from build123d import *

# Parameters (mm, degrees)
SKETCH3_W                = 19.05
SKETCH3_H                = 19.05
SKETCH3_W_2              = 16.002
SKETCH3_H_2              = 16.002
BOSS_EXTRUDE1_DEPTH      = 25.4
BOSS_EXTRUDE1_DEPTH_BACK = 25.4
FILLET1_R                = 1.6002
SKETCH5_W                = 19.784949474
SKETCH5_H                = 25.4
CUT_EXTRUDE1_DEPTH       = 17.4625
SKETCH7_R                = 2.15265
CUT_EXTRUDE2_DEPTH       = 12.7
SKETCH6_R                = 2.15265
CUT_EXTRUDE3_DEPTH       = 2.524
SKETCH9_R                = 2.15265
CUT_EXTRUDE5_DEPTH       = 6.35
SKETCH10_R               = 2.15265
CUT_EXTRUDE6_DEPTH       = 20.05


with BuildPart() as part:
    # Sketch3 → Boss-Extrude1 (new body, two sides)
    with BuildSketch(Plane.XY) as boss_extrude1_sk:
        Rectangle(SKETCH3_W, SKETCH3_H)
        Rectangle(SKETCH3_W_2, SKETCH3_H_2, mode=Mode.SUBTRACT)
    extrude(amount=BOSS_EXTRUDE1_DEPTH)
    extrude(boss_extrude1_sk.sketch, amount=-BOSS_EXTRUDE1_DEPTH_BACK)

    # Fillet1
    fillet1_edges = [part.edges().sort_by_distance(p)[0] for p in [
        (8.001, -8.001, 0),
        (8.001, 8.001, 0),
        (-8.001, 8.001, 0),
        (-8.001, -8.001, 0),
        (9.525, -9.525, 0),
        (-9.525, -9.525, 0),
        (-9.525, 9.525, 0),
        (9.525, 9.525, 0),
    ]]
    fillet(fillet1_edges, radius=FILLET1_R)

    # Sketch5 → Cut-Extrude1 (cut)
    with BuildSketch(Plane(origin=(0, 9.525, 0), x_dir=(1, 0, 0), z_dir=(0, 1, 0))):
        with Locations((1.967674737, 0)):
            Rectangle(SKETCH5_W, SKETCH5_H)
    extrude(amount=-CUT_EXTRUDE1_DEPTH, mode=Mode.SUBTRACT)

    # Sketch7 → Cut-Extrude2 (cut)
    with BuildSketch(Plane(origin=(0, 9.525, 0), x_dir=(1, 0, 0), z_dir=(0, 1, 0))):
        with Locations((0, 19.05)):
            Circle(SKETCH7_R)
        with Locations((2.54, 0)):
            Circle(SKETCH7_R)
        with Locations((0, -19.05)):
            Circle(SKETCH7_R)
    extrude(amount=-CUT_EXTRUDE2_DEPTH, mode=Mode.SUBTRACT)

    # Sketch6 → Cut-Extrude3 (cut, through all)
    with BuildSketch(Plane(origin=(0, -8.001, 0), x_dir=(1, 0, 0), z_dir=(0, 1, 0))):
        with Locations((2.54, 0)):
            Circle(SKETCH6_R)
    extrude(amount=-CUT_EXTRUDE3_DEPTH, mode=Mode.SUBTRACT)

    # Sketch9 → Cut-Extrude5 (cut)
    with BuildSketch(Plane(origin=(9.525, 0, 0), x_dir=(0, 0, -1), z_dir=(1, 0, 0))):
        with Locations((-19.05, 0)):
            Circle(SKETCH9_R)
        with Locations((19.05, 0)):
            Circle(SKETCH9_R)
    extrude(amount=-CUT_EXTRUDE5_DEPTH, mode=Mode.SUBTRACT)

    # Sketch10 → Cut-Extrude6 (cut, through all)
    with BuildSketch(Plane(origin=(9.525, 0, 0), x_dir=(0, 0, -1), z_dir=(1, 0, 0))):
        with Locations((0, 2.54)):
            Circle(SKETCH10_R)
    extrude(amount=-CUT_EXTRUDE6_DEPTH, mode=Mode.SUBTRACT)


solid = part.part
The model under review builds one solid part; all positions refer to its coordinate system, in mm. A direction names the side the tool comes from. Give positions to 0.01 mm unless a question says otherwise; leave off trailing zeros. Loops run counter-clockwise (first coordinate to the right, second up) from the corner with the lowest first, then second, coordinate; pieces in that order, holes last. Notation, with made-up numbers: (52, 29.5) -> (94, 29.5) arc R21 cw to (94, 62.5) -> close; hole circle Ø7 at (4.25, 15.25). An arc over 180 degrees is marked (long way). Write each question's results on one line, items separated by ' | '.
1) Draft analysis for pull direction Y (two halves, no side actions). For faces 6 (the face through (-0.47, 8.77, 21.15)), 7 (the face through (9.07, -9.04, 0.36)), 8 (the face through (-8.001, 0, 0)), state which applies: pulls with the +Y half, pulls with the -Y half, needs draft (parallel to the pull), parting line crosses it, or undercut.
Conclusion:
face 6: needs draft | face 7: pulls with the -Y half | face 8: undercut
2) Take a section at D-D, the plane z = -19.05. Give the boundary of the cut face in (x, y) (3 decimals), plus the area to 3 significant figures.
Conclusion:
outline: (-9.525, -7.925) arc R1.6 ccw to (-7.925, -9.525) -> (7.925, -9.525) arc R1.6 ccw to (9.525, -7.925) -> (9.525, -2.153) -> (8.001, -2.153) -> (8.001, -6.401) arc R1.6 cw to (6.401, -8.001) -> (-6.401, -8.001) arc R1.6 cw to (-8.001, -6.401) -> (-8.001, 6.401) arc R1.6 cw to (-6.401, 8.001) -> (-2.153, 8.001) -> (-2.153, 9.525) -> (-7.925, 9.525) arc R1.6 ccw to (-9.525, 7.925) -> close; (2.153, 8.001) -> (6.401, 8.001) arc R1.6 cw to (8.001, 6.401) -> (8.001, 2.153) -> (9.525, 2.153) -> (9.525, 7.925) arc R1.6 ccw to (7.925, 9.525) -> (2.153, 9.525) -> close | area: 93.7 mm^2
3) Take a section at A-A, the plane x = -5.5. Give the boundary of the cut face in (y, z) (3 decimals).
Conclusion:
outline: (-9.525, -25.4) -> (-8.001, -25.4) -> (-8.001, 25.4) -> (-9.525, 25.4) -> close; (8.001, -25.4) -> (9.525, -25.4) -> (9.525, -12.7) -> (8.001, -12.7) -> close; (8.001, 12.7) -> (9.525, 12.7) -> (9.525, 25.4) -> (8.001, 25.4) -> close
4) Insertion check: pin 1 Ø7 at (y, z) = (2.54, 0) entering from +X; pin 2 Ø1.3 at (y, z) = (7.5, 0) entering from +X; pin 3 Ø10 at (x, z) = (1.5, -5) entering from +Y; pin 4 Ø0.8 at (x, y) = (-7.5, -7.5) entering from +Z. Each pin has a flat end and moves straight along its axis. Give the tip position at first contact, or say it passes through.
Conclusion:
pin 1: stops at x = -8 | pin 2: stops at x = -7.92 | pin 3: stops at y = -8 | pin 4: stops at z = 25.4
5) For line 1 along Z through (x, y) = (0, 9.2); line 2 along Y through (x, z) = (-3.5, -22) (3 decimals), list the stretches that pass through material, from the lowest coordinate up. Write a range as from..to.
Conclusion:
line 1: z = -25.4..-21.2, -16.9..-12.7, 12.7..16.9, 21.2..25.4 | line 2: y = -9.525..-8.001, 8.001..9.525
6) Take a section at C-C, the plane z = 14. Give the boundary of the cut face in (x, y) (3 decimals).
Conclusion:
outline: (-9.525, -7.925) arc R1.6 ccw to (-7.925, -9.525) -> (7.925, -9.525) arc R1.6 ccw to (9.525, -7.925) -> (9.525, 7.925) arc R1.6 ccw to (7.925, 9.525) -> (-7.925, 9.525) arc R1.6 ccw to (-9.525, 7.925) -> close; hole (-8.001, -6.401) arc R1.6 ccw to (-6.401, -8.001) -> (6.401, -8.001) arc R1.6 ccw to (8.001, -6.401) -> (8.001, 6.401) arc R1.6 ccw to (6.401, 8.001) -> (-6.401, 8.001) arc R1.6 ccw to (-8.001, 6.401) -> close
7) Tool access review of faces 1 (the face through (-7.7, -7.6, 12.7)), 2 (the face through (-1.9, 9.525, -17.5)), 3 (the face through (8.8, 0.1, 21.2)), 4 (the face through (8.001, 0, 22)), 5 (the face through (9.07, 9.04, -19.14)): name each direction out of +Z, -Z, +X, -X, +Y, -Y from which nothing blocks a thin tool from reaching the whole face with its end or side.
Conclusion:
face 1: +X, +Y | face 2: +Z, -Z, +X, -X, +Y | face 3: +X | face 4: +Z, -Z | face 5: +Z, -Z, +X, +Y
